```python
from build123d import *

# Parameters (mm, degrees)
SKETCH1_R           = 2.999994
BOSS_EXTRUDE1_DEPTH = 6.858
SKETCH2_W           = 50.8
SKETCH2_H           = 9.525
BOSS_EXTRUDE2_DEPTH = 24.892
CUT_EXTRUDE1_DEPTH  = 24.892
SKETCH4_W           = 6.35
SKETCH4_H           = 18.373928642
CUT_EXTRUDE2_DEPTH  = 58.166


with BuildPart() as part:
    # Sketch1 → Boss-Extrude1 (new body)
    with BuildSketch(Plane(origin=(0, 0, 0), x_dir=(1, 0, 0), z_dir=(0, 1, 0))):
        with BuildLine():
            Line((22.86, -25.4), (-22.86, -25.4))
            ThreePointArc((-22.86, -25.4), (-24.656051224, -24.656051224), (-25.4, -22.86))
            Line((-25.4, -22.86), (-25.4, 22.86))
            ThreePointArc((-25.4, 22.86), (-24.656051224, 24.656051224), (-22.86, 25.4))
            Line((-22.86, 25.4), (22.86, 25.4))
            ThreePointArc((22.86, 25.4), (24.656051224, 24.656051224), (25.4, 22.86))
            Line((25.4, 22.86), (25.4, -22.86))
            ThreePointArc((25.4, -22.86), (24.656051224, -24.656051224), (22.86, -25.4))
        make_face()
        with Locations(Location((-18.499963, 18.499963, 0), (0, 0, 270))):
            Circle(SKETCH1_R, mode=Mode.SUBTRACT)
        with Locations(Location((18.499963, 18.499963, 0), (0, 0, 270))):
            Circle(SKETCH1_R, mode=Mode.SUBTRACT)
        with Locations(Location((18.499963, -18.499963, 0), (0, 0, 270))):
            Circle(SKETCH1_R, mode=Mode.SUBTRACT)
        with Locations(Location((-18.499963, -18.499963, 0), (0, 0, 270))):
            Circle(SKETCH1_R, mode=Mode.SUBTRACT)
    extrude(amount=BOSS_EXTRUDE1_DEPTH)

    # Sketch2 → Boss-Extrude2 (add)
    with BuildSketch(Plane(origin=(0, 6.858, 0), x_dir=(1, 0, 0), z_dir=(0, 1, 0))):
        with Locations((0, -4.7625)):
            Rectangle(SKETCH2_W, SKETCH2_H)
        with Locations((0, 4.7625)):
            Rectangle(SKETCH2_W, SKETCH2_H)
    extrude(amount=BOSS_EXTRUDE2_DEPTH)

    # Sketch3 → Cut-Extrude1 (cut)
    with BuildSketch(Plane.XY.offset(9.525)):
        with BuildLine():
            ThreePointArc((6.35, 16.103217479), (4.490128061, 20.593345539), (0, 22.453217479))
            Line((0, 22.453217479), (0, 9.753217479))
            ThreePointArc((0, 9.753217479), (4.490128061, 11.613089418), (6.35, 16.103217479))
        make_face()
        with BuildLine():
            Line((0, 9.753217479), (0, 22.453217479))
            ThreePointArc((0, 22.453217479), (-6.35, 16.103217479), (0, 9.753217479))
        make_face()
        with BuildLine():
            Line((25.4, 31.75), (0, 31.75))
            Line((0, 31.75), (0, 25.231928642))
            ThreePointArc((0, 25.231928642), (15.674511585, 20.156909879), (25.4, 6.858))
            Line((25.4, 6.858), (25.4, 31.75))
        make_face()
        with BuildLine():
            Line((0, 25.231928642), (0, 31.75))
            Line((0, 31.75), (-25.4, 31.75))
            Line((-25.4, 31.75), (-25.4, 6.858))
            ThreePointArc((-25.4, 6.858), (-15.674511585, 20.156909879), (0, 25.231928642))
        make_face()
    extrude(amount=-CUT_EXTRUDE1_DEPTH, mode=Mode.SUBTRACT)

    # Sketch4 → Cut-Extrude2 (cut)
    with BuildSketch(Plane.ZY.offset(25.4)):
        with Locations((0, 16.044964321)):
            Rectangle(SKETCH4_W, SKETCH4_H)
    extrude(amount=-CUT_EXTRUDE2_DEPTH, mode=Mode.SUBTRACT)


solid = part.part
```
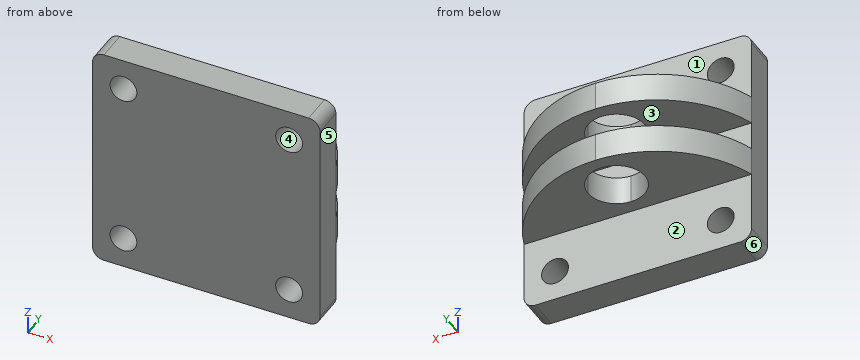
CAD build for the part. Positions are in the model's coordinates, mm. Face numbers are marked on the shaded views. A direction names the side the tool comes from. Round coordinates to 2 decimals unless told otherwise and drop trailing zeros. Order: outer loops, then holes, each group sorted by start corner. A loop starts at its lowest first (then second) coordinate and runs counter-clockwise, first axis right, second up. Notation, with made-up numbers: (85, 23.25) -> (142, 23.25) arc R29 cw to (142, 50.25) -> close; hole circle Ø2 at (-37.75, 21.25). An arc over 180 degrees is marked (long way). One line per question, with ' | ' between items.
Q1. Which spindle directions (+Z, -Z, +X, -X, +Y, -Y) get a long thin tool onto all of the face, cutting with end or side? Do the marked faces 1, 2 and 3. Say none if no direction does.
Completed:
face 1: +Z, +X, -X, +Y | face 2: -Z, +X, -X, +Y | face 3: +X, -X, +Y
Q2. Slice it at A-A (y = 17.75). Write the cut outline in (x, z) (3 decimals).
Completed:
outline: (-18.553, -9.525) -> (-6.133, -9.525) -> (-6.133, -3.175) -> (-18.553, -3.175) -> close; (-18.553, 3.175) -> (-6.133, 3.175) -> (-6.133, 9.525) -> (-18.553, 9.525) -> close; (6.133, -9.525) -> (18.553, -9.525) -> (18.553, -3.175) -> (6.133, -3.175) -> close; (6.133, 3.175) -> (18.553, 3.175) -> (18.553, 9.525) -> (6.133, 9.525) -> close
Q3. Two-plate mould, pull along Z, no slides. Class the marked faces 4, 5 and 6: released by +Z, released by -Z, zero draft, split by the parting line, or undercut.
Completed:
face 4: undercut | face 5: zero draft | face 6: released by -Z
Q4. Drop flat-ended pins along their axis: pin 1 (9.5 mm diameter, centred on x = -18.5, z = 18.5, fed in from +Y); pin 2 (5.5 mm diameter, centred on x = 18.5, z = 18.5, fed in from -Y); pin 3 (8 mm diameter, centred on x = -11.5, y = 22, fed in from -Z) (3 decimals); pin 4 (8 mm diameter, centred on x = 4.5, y = 22, fed in from +Z) (3 decimals). Give the stop position or say it passes through.
Completed:
pin 1: stops at y = 6.86 | pin 2: passes through | pin 3: stops at z = -9.525 | pin 4: stops at z = 9.525
Q5. Probe probe 1 along Z at (x, y) = (13, 14.5) (3 decimals); probe 2 along X at (y, z) = (6.75, 20.5); probe 3 along Y at (x, z) = (8, -11.5). List the from-to ranges inside material, lowest first.
Completed:
probe 1: z = -9.525 to -3.175, 3.175 to 9.525 | probe 2: x = -25.4 to -20.74, -16.26 to 16.26, 20.74 to 25.4 | probe 3: y = 0 to 6.86
Q6. Slice it at C-C (y = 8.5). Write the cut outline in (x, z) (3 decimals), then the cut area to 3 significant figures.
Completed:
outline: (-24.799, -9.525) -> (24.799, -9.525) -> (24.799, -3.175) -> (-24.799, -3.175) -> close; (-24.799, 3.175) -> (24.799, 3.175) -> (24.799, 9.525) -> (-24.799, 9.525) -> close | area: 630 mm^2
Q7. Slice it at D-D (x = 8). Write the cut outline in (y, z) (3 decimals), then the cut area to 3 significant figures.
Completed:
outline: (0, -25.4) -> (6.858, -25.4) -> (6.858, -9.525) -> (24.007, -9.525) -> (24.007, -3.175) -> (6.858, -3.175) -> (6.858, 3.175) -> (24.007, 3.175) -> (24.007, 9.525) -> (6.858, 9.525) -> (6.858, 25.4) -> (0, 25.4) -> close | area: 566 mm^2
Q8. Slice it at B-B (z = 17.5). Write the cut outline in (x, y), then the cut area to 3 significant figures.
Completed:
outline: (-25.4, 0) -> (-21.33, 0) -> (-21.33, 6.86) -> (-25.4, 6.86) -> close; (-15.67, 0) -> (15.67, 0) -> (15.67, 6.86) -> (-15.67, 6.86) -> close; (21.33, 0) -> (25.4, 0) -> (25.4, 6.86) -> (21.33, 6.86) -> close | area: 271 mm^2
